CAD build for the part. Positions are in the model's coordinates, mm. Face numbers are marked on the shaded views. Give positions to 0.01 mm unless a question says otherwise; leave off trailing zeros. Order: outer loops, then holes, each group sorted by start corner. A loop starts at its lowest first (then second) coordinate and runs counter-clockwise, first axis right, second up.
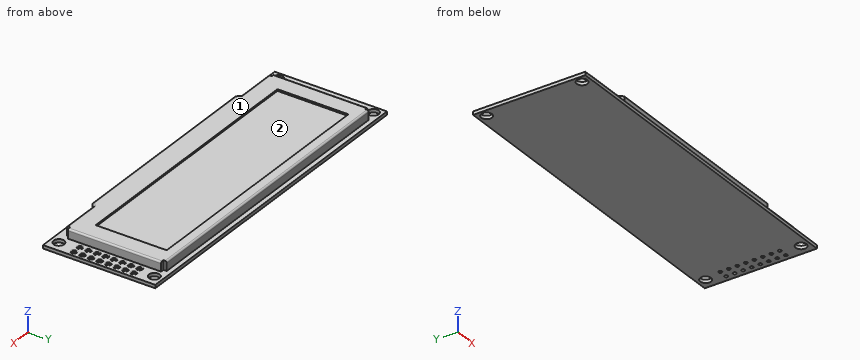
from build123d import *

# Parameters (mm, degrees)
SKETCH_1_W          = 100.5
SKETCH_1_H          = 33.5
SKETCH_1_R          = 1.6
EXTRUDE_1_DEPTH     = 1
EXTRUDE_2_DEPTH     = 2.8
FILLET_1_R          = 0.5
SKETCH_3_W          = 78.8
SKETCH_3_H          = 21.18
CUT_EXTRUDE_1_DEPTH = 0.5
SKETCH_4_R          = 0.9
EXTRUDE_3_DEPTH     = 0.1
SKETCH_5_R          = 0.5
CUT_EXTRUDE_2_DEPTH = 2.1


with BuildPart() as part:
    # Эскиз1 → Бобышка-Вытянуть1 (new body)
    with BuildSketch(Plane.XY):
        Rectangle(SKETCH_1_W, SKETCH_1_H)
        with Locations((-48, 14.25)):
            Circle(SKETCH_1_R, mode=Mode.SUBTRACT)
        with Locations((47, 14.25)):
            Circle(SKETCH_1_R, mode=Mode.SUBTRACT)
        with Locations((47, -14.25)):
            Circle(SKETCH_1_R, mode=Mode.SUBTRACT)
        with Locations((-48, -14.25)):
            Circle(SKETCH_1_R, mode=Mode.SUBTRACT)
    extrude(amount=EXTRUDE_1_DEPTH)

    # Эскиз2 → Бобышка-Вытянуть2 (add)
    with BuildSketch(Plane.XY.offset(1)):
        Polygon((43.25, 15.35), (-44.25, 15.35), (-44.25, 14.35), (-45.25, 14.35), (-45.25, -13.45), (-44.25, -13.45), (-44.25, -14.45), (-32.65, -14.45), (-31.5, -15.6), (30.5, -15.6), (31.65, -14.45), (43.25, -14.45), (43.25, -13.45), (44.25, -13.45), (44.25, 14.35), (43.25, 14.35), align=None)
    extrude(amount=EXTRUDE_2_DEPTH)

    # Скругление1
    fillet_1_edges = [part.edges().sort_by_distance(p)[0] for p in [
        (-45.25, 0.45, 3.8),
        (-38.45, -14.45, 3.8),
        (-32.075, -15.025, 3.8),
        (-0.5, -15.6, 3.8),
        (31.075, -15.025, 3.8),
        (37.45, -14.45, 3.8),
        (44.25, 0.45, 3.8),
        (-0.5, 15.35, 3.8),
    ]]
    fillet(fillet_1_edges, radius=FILLET_1_R)

    # Эскиз3 → Вырез-Вытянуть1 (cut)
    with BuildSketch(Plane.XY.offset(3.8)):
        with Locations((-0.5, 1.76)):
            Rectangle(SKETCH_3_W, SKETCH_3_H)
    extrude(amount=-CUT_EXTRUDE_1_DEPTH, mode=Mode.SUBTRACT)

    # Эскиз4 → Бобышка-Вытянуть3 (add)
    with BuildSketch(Plane.XY.offset(1)):
        with Locations((48.5, -8.64)):
            Circle(SKETCH_4_R)
        with Locations((45.96, -8.64)):
            Circle(SKETCH_4_R)
        with Locations((45.96, -6.1)):
            Circle(SKETCH_4_R)
        with Locations((45.96, -3.56)):
            Circle(SKETCH_4_R)
        with Locations((45.96, -1.02)):
            Circle(SKETCH_4_R)
        with Locations((45.96, 1.52)):
            Circle(SKETCH_4_R)
        with Locations((45.96, 4.06)):
            Circle(SKETCH_4_R)
        with Locations((45.96, 6.6)):
            Circle(SKETCH_4_R)
        with Locations((45.96, 9.14)):
            Circle(SKETCH_4_R)
        with Locations((48.5, -6.1)):
            Circle(SKETCH_4_R)
        with Locations((48.5, -3.56)):
            Circle(SKETCH_4_R)
        with Locations((48.5, -1.02)):
            Circle(SKETCH_4_R)
        with Locations((48.5, 1.52)):
            Circle(SKETCH_4_R)
        with Locations((48.5, 4.06)):
            Circle(SKETCH_4_R)
        with Locations((48.5, 6.6)):
            Circle(SKETCH_4_R)
        with Locations((48.5, 9.14)):
            Circle(SKETCH_4_R)
    extrude(amount=EXTRUDE_3_DEPTH)

    # Эскиз5 → Вырез-Вытянуть2 (cut, through all)
    with BuildSketch(Plane.XY.offset(1.1)):
        with Locations((48.5, -8.64)):
            Circle(SKETCH_5_R)
        with Locations((45.96, -8.64)):
            Circle(SKETCH_5_R)
        with Locations((45.96, -6.1)):
            Circle(SKETCH_5_R)
        with Locations((45.96, -3.56)):
            Circle(SKETCH_5_R)
        with Locations((45.96, -1.02)):
            Circle(SKETCH_5_R)
        with Locations((45.96, 1.52)):
            Circle(SKETCH_5_R)
        with Locations((45.96, 4.06)):
            Circle(SKETCH_5_R)
        with Locations((45.96, 6.6)):
            Circle(SKETCH_5_R)
        with Locations((45.96, 9.14)):
            Circle(SKETCH_5_R)
        with Locations((48.5, -6.1)):
            Circle(SKETCH_5_R)
        with Locations((48.5, -3.56)):
            Circle(SKETCH_5_R)
        with Locations((48.5, -1.02)):
            Circle(SKETCH_5_R)
        with Locations((48.5, 1.52)):
            Circle(SKETCH_5_R)
        with Locations((48.5, 4.06)):
            Circle(SKETCH_5_R)
        with Locations((48.5, 6.6)):
            Circle(SKETCH_5_R)
        with Locations((48.5, 9.14)):
            Circle(SKETCH_5_R)
    extrude(amount=-CUT_EXTRUDE_2_DEPTH, mode=Mode.SUBTRACT)


solid = part.part
1. Mould opens along Y. For the marked faces 1 and 2 say: released by +Y, released by -Y, zero draft, split by the parting line, or undercut.
2. Saw through at D-D on z = 1.7. Give the cut face in (x, y), plus the area to 3 significant figures.
3. Saw through at B-B on x = -4. Give the cut face in (y, z), plus the area to 3 significant figures.
4. Pin check, flat tips, straight feed: P1, Ø2, axis at x = 48, y = 1.5, coming from the +Z side; P2, Ø4, axis at x = 47, y = 14.25, coming from the +Z side; P3, Ø2, axis at y = 7.5, z = 3.5, coming from the +X side. Stop position of each tip, or through.
5. Wall check: line 1 (Y direction, x = -43.5, z = 3.4); line 2 (X direction, y = -11, z = 2.2); line 3 (Y direction, x = 11, z = 1.1). Give the ranges that are in metal, low to high.
6. Saw through at C-C on y = -11. Give the cut face in (x, z).
7. Saw through at A-A on x = -48. Give the cut face in (y, z).
Reported:
1. face 1: zero draft
1. face 2: undercut
2. outline: (-45.25, -13.45) - (-44.25, -13.45) - (-44.25, -14.45) - (-32.65, -14.45) - (-31.5, -15.6) - (30.5, -15.6) - (31.65, -14.45) - (43.25, -14.45) - (43.25, -13.45) - (44.25, -13.45) - (44.25, 14.35) - (43.25, 14.35) - (43.25, 15.35) - (-44.25, 15.35) - (-44.25, 14.35) - (-45.25, 14.35) - close
2. area: 2,740 mm2
3. outline: (-16.75, 0) - (16.75, 0) - (16.75, 1) - (15.35, 1) - (15.35, 3.3) arc R0.5 ccw to (14.85, 3.8) - (12.35, 3.8) - (12.35, 3.3) - (-8.83, 3.3) - (-8.83, 3.8) - (-15.1, 3.8) arc R0.5 ccw to (-15.6, 3.3) - (-15.6, 1) - (-16.75, 1) - close
3. area: 109 mm2
4. P1: stops at z = 1.1
4. P2: stops at z = 1
4. P3: stops at x = 44.25
5. line 1: y = -14.44 to 15.34
5. line 2: x = -45.25 to 44.25
5. line 3: y = -15.6 to 15.35
6. outline: (-50.25, 0) - (50.25, 0) - (50.25, 1) - (44.25, 1) - (44.25, 3.3) arc R0.5 ccw to (43.75, 3.8) - (-44.75, 3.8) arc R0.5 ccw to (-45.25, 3.3) - (-45.25, 1) - (-50.25, 1) - close
7. outline: (-16.75, 0) - (-15.85, 0) - (-15.85, 1) - (-16.75, 1) - close; (-12.65, 0) - (12.65, 0) - (12.65, 1) - (-12.65, 1) - close; (15.85, 0) - (16.75, 0) - (16.75, 1) - (15.85, 1) - close
